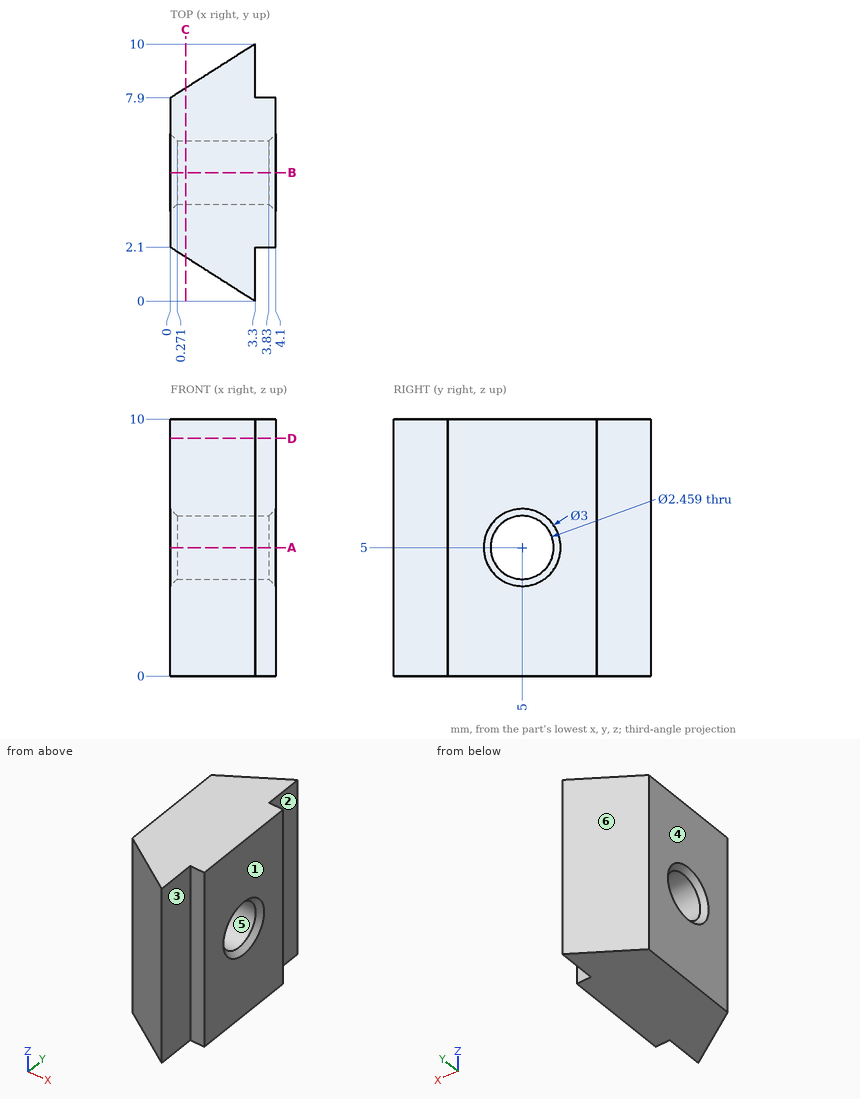
Study the drawing (mm; zero at the part's minimum x, y, z) and answer. A direction names the side the tool comes from. Give positions to 0.01 mm unless a question says otherwise; leave off trailing zeros. Loops run counter-clockwise (first coordinate to the right, second up) from the corner with the lowest first, then second, coordinate; pieces in that order, holes last. Notation, with made-up numbers: (73, 59.25) - (80, 59.25) arc R26 cw to (80, 92.25) - close; hole circle Ø11 at (24.25, -21). An arc over 180 degrees is marked (long way). Return JSON: item names as keys, results as strings. Group by question number.
1. Find section B-B (y = 5). Write down the section's boundary in (x, z).
2. Find section C-C (x = 0.6). Write down the section's boundary in (y, z).
3. Find section D-D (z = 9.25). Write down the section's boundary in (x, y).
4. Given pin 1 Ø0.6 at (y, z) = (1, 5.5) entering from +X; pin 2 Ø1 at (y, z) = (5, 5.5) entering from -X, each flat-ended and moving along its own axis, determine where each tip first touches the part or whether it passes through.
5. Which of the six approach directions +Z, -Z, +X, -X, +Y, -Y give full straight-line access (tool end or side, diameter ignored) to the marked faces 1, 2 and 3?
6. Determine the mould class of the marked faces 4, 5 and 6 for opening direction Y: pulls with the +Y half, pulls with the -Y half, needs draft (parallel to the pull), parting line crosses it, or undercut.
7. Find section A-A (z = 5). Write down the section's boundary in (x, y), then the cut area to 3 significant figures.
8. Straight lines are drawn through the part: line 1 (Z direction, x = 1.65, y = 5); line 2 (Y direction, x = 1.35, z = 5.75) (1 decimal); line 3 (Y direction, x = 2.85, z = 5.5) (1 decimal). For each, find the intervals that lie inside material, in ascending order. Write a range as [from, to].
Verdict:
{
 "1": {"outline": "(0, 0) - (4.1, 0) - (4.1, 3.5) - (3.83, 3.77) - (0.27, 3.77) - (0, 3.5) - close; (0, 6.5) - (0.27, 6.23) - (3.83, 6.23) - (4.1, 6.5) - (4.1, 10) - (0, 10) - close"},
 "2": {"outline": "(1.72, 0) - (8.28, 0) - (8.28, 10) - (1.72, 10) - close; hole circle Ø2.46 at (5, 5)"},
 "3": {"outline": "(0, 2.1) - (3.3, 0) - (3.3, 2.1) - (4.1, 2.1) - (4.1, 7.9) - (3.3, 7.9) - (3.3, 10) - (0, 7.9) - close"},
 "4": {"pin 1": "stops at x = 3.3", "pin 2": "passes through"},
 "5": {"face 1": "+Z, -Z, +X, +Y, -Y", "face 2": "+Z, -Z, +X, +Y", "face 3": "+Z, -Z, +X, -Y"},
 "6": {"face 4": "needs draft", "face 5": "undercut", "face 6": "pulls with the +Y half"},
 "7": {"outline": "(0, 2.1) - (3.3, 0) - (3.3, 2.1) - (4.1, 2.1) - (4.1, 3.5) - (3.83, 3.77) - (0.27, 3.77) - (0, 3.5) - close; (0, 6.5) - (0.27, 6.23) - (3.83, 6.23) - (4.1, 6.5) - (4.1, 7.9) - (3.3, 7.9) - (3.3, 10) - (0, 7.9) - close", "area": "20.5 mm^2"},
 "8": {"line 1": "z = [0, 3.77], [6.23, 10]", "line 2": "y = [1.2, 4], [6, 8.8]", "line 3": "y = [0.3, 3.9], [6.1, 9.7]"}
}
